Can you work these out from the model? Positions are in its coordinate system, mm. Face numbers are marked on the shaded views. A direction names the side the tool comes from. Give positions to 0.01 mm unless a question says otherwise; leave off trailing zeros. Order: outer loops, then holes, each group sorted by start corner. A loop starts at its lowest first (then second) coordinate and runs counter-clockwise, first axis right, second up.
Item 1: Which directions (+Z, -Z, +X, -X, +Y, -Y) give clear straight access to the entire face, cutting with the end or side of a thin tool? Please do the marked faces 3 and 4.
Item 2: I want a section at C-C, the plane z = 3.95. Write out the boundary of the cut face in (x, y).
Item 3: I want a section at D-D, the plane y = -15. Write out the boundary of the cut face in (x, z).
Item 4: If we mould it in two halves opening along X, with no side actions, what happens to the marked faces 1 and 2? For each: +X half, -X half, draft (parallel to the pull), parting line (faces both ways), or undercut.
Item 5: I'm going to push flat-ended pins straight in: pin 1 Ø3 at (x, y) = (7.5, 19.5) entering from -Z; pin 2 Ø2.5 at (y, z) = (-22.5, 2.5) entering from -X; pin 3 Ø2.5 at (y, z) = (17.5, 2) entering from -X; pin 4 Ø2.5 at (x, z) = (29.5, 1.5) entering from +Y. Where does each tip first touch, or does it pass through?
Item 6: If I drill on line 1 along Y through (x, z) = (0, 2.8); line 2 along X through (y, z) = (-22, 1.85); line 3 along X through (y, z) = (-8, 3.6), over which ranges is the centre line in solid material (lowest first)?
Item 7: I want a section at A-A, the plane x = 0. Write out the boundary of the cut face in (y, z), then the cut area to 3 significant figures.
Item 8: I want a section at B-B, the plane y = 0. Write out the boundary of the cut face in (x, z), then the cut area to 3 significant figures.
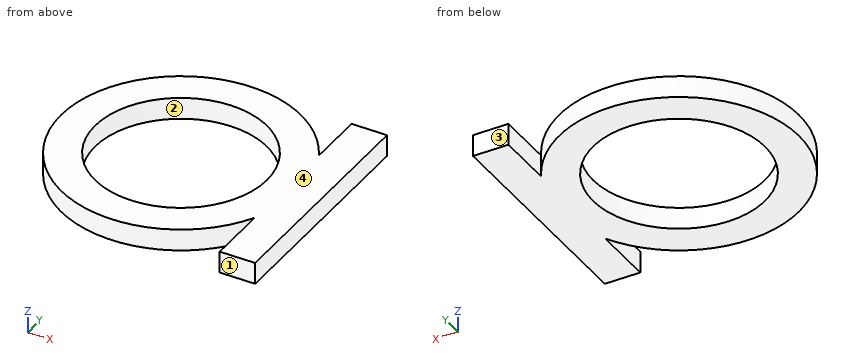
```python
from build123d import *

# Parameters (mm, degrees)
F0_R     = 27.496488
F1_DEPTH = 5
F2_R     = 19.711681
F3_DEPTH = 5
F4_W     = 8.140551
F4_H     = 52.797299
F5_DEPTH = 5


with BuildPart() as f1:
    # F0 (on Top) → F1 (new body)
    with BuildSketch(Plane.XY):
        Circle(F0_R)
    extrude(amount=F1_DEPTH)

    # F2 (on face) → F3 (cut)
    with BuildSketch(Plane.XY.offset(5)):
        Circle(F2_R)
    extrude(amount=-F3_DEPTH, mode=Mode.SUBTRACT)

    # F4 (on Top) → F5 (join)
    with BuildSketch(Plane.XY):
        with Locations((28.375639, -0.465175)):
            Rectangle(F4_W, F4_H)
    extrude(amount=F5_DEPTH)


solid = f1.part
```
Results list:
1. face 3: +Z, -Z, +X, +Y
1. face 4: +Z, +X, -X, +Y, -Y
2. outline: (24.31, -26.86) - (32.45, -26.86) - (32.45, 25.93) - (24.31, 25.93) - (24.31, 12.86) arc R27.5 ccw (long way) to (24.31, -12.86) - close; hole circle Ø39.42 at (0, 0)
3. outline: (-23.04, 0) - (-12.79, 0) - (-12.79, 5) - (-23.04, 5) - close; (12.79, 0) - (23.04, 0) - (23.04, 5) - (12.79, 5) - close; (24.31, 0) - (32.45, 0) - (32.45, 5) - (24.31, 5) - close
4. face 1: draft
4. face 2: undercut
5. pin 1: stops at z = 0
5. pin 2: stops at x = -17.45
5. pin 3: stops at x = -22.18
5. pin 4: stops at y = 25.93
6. line 1: y = -27.5 to -19.71, 19.71 to 27.5
6. line 2: x = -16.49 to 16.49, 24.31 to 32.45
6. line 3: x = -26.31 to -18.02, 18.02 to 32.45
7. outline: (-27.5, 0) - (-19.71, 0) - (-19.71, 5) - (-27.5, 5) - close; (19.71, 0) - (27.5, 0) - (27.5, 5) - (19.71, 5) - close
7. area: 77.8 mm2
8. outline: (-27.5, 0) - (-19.71, 0) - (-19.71, 5) - (-27.5, 5) - close; (19.71, 0) - (32.45, 0) - (32.45, 5) - (19.71, 5) - close
8. area: 103 mm2
